Work out the finished part from the listing and answer in its coordinate system (mm). Face numbers are marked on the shaded views. A direction names the side the tool comes from. Coordinates: 2 decimals unless noted, no trailing zeros. Write each loop counter-clockwise with the first axis right and the second up, starting at its lowest first coordinate (ties: lowest second). Pieces come first, ordered by that corner, then holes. Notation, with made-up numbers: (82.25, 1) - (99.25, 1) arc R13 ccw to (99.25, 26) - close; hole circle Ø9 at (-1.75, 41.25). An arc over 180 degrees is marked (long way). Use a Markdown table: item, result. Add a question column.
(1) The part is cut by section B-B, the plane y = 40. Give the vertices of the cut face in (x, z), then the cut area to 3 significant figures.
(2) A tool of negligible diameter and unlimited length cuts with its end or side. For the marked faces 4, 5, 6 and 7, from which of +Z, -Z, +X, -X, +Y, -Y can it reach the whole face along a straight path? Write none if from no direction.
(3) The part is cut by section D-D, the plane z = 34.5. Give the vertices of the cut face in (x, y), then the cut area to 3 significant figures.
(4) Find the intervals of material crossed by line 1 (Y direction, x = 4, z = -30); line 2 (Z direction, x = 54.5, y = 61.5); line 3 (X direction, y = 60, z = -11), in increasing order. Write a range as from..to.
(5) For a pull along Y with two mould halves and no side action, classify the marked faces 1, 2 and 3 as released by +Y, released by -Y, zero draft, split by the parting line, or undercut.
(6) The part is cut by section C-C, the plane x = 24. Give the vertices of the cut face in (y, z), then the cut area to 3 significant figures.
(7) Given pin 1 Ø18.5 at (x, z) = (7.5, 30.5) entering from -Y; pin 2 Ø12 at (y, z) = (37.5, 26.5) entering from +X; pin 3 Ø13.5 at (x, z) = (6, 24) entering from +Y; pin 4 Ø10 at (x, z) = (26.5, 32) entering from -Y, each flat-ended and moving along its own axis, determine where each tip first touches the part or whether it passes through.
(8) The part is cut by section A-A, the plane z = -30. Give the vertices of the cut face in (x, y), then the cut area to 3 significant figures.
from build123d import *

# Parameters (mm, degrees)
BOSS_EXTRUDE1_DEPTH = 80
CUT_EXTRUDE1_DEPTH  = 80
SKETCH4_R           = 6
CUT_EXTRUDE4_DEPTH  = 80
BOSS_EXTRUDE2_DEPTH = 17
SKETCH9_R           = 7.5
CUT_EXTRUDE5_DEPTH  = 17
FILLET2_R           = 10
FILLET3_R           = 10


with BuildPart() as part:
    # Sketch1 → Boss-Extrude1 (new body)
    with BuildSketch(Plane(origin=(0, 0, 0), x_dir=(1, 0, 0), z_dir=(0, 1, 0))):
        Polygon((0, 0), (58, 0), (58, 13), (17, 13), (17, 47), (58, 47), (58, 60), (0, 60), align=None)
    extrude(amount=BOSS_EXTRUDE1_DEPTH)

    # Sketch2 → Cut-Extrude1 (cut)
    with BuildSketch(Plane.XY):
        with BuildLine():
            Line((38.781649875, 11), (38.781649875, 63))
            ThreePointArc((38.781649875, 63), (45, 69.218350125), (51.218350125, 63))
            Line((51.218350125, 63), (51.218350125, 11))
            ThreePointArc((51.218350125, 11), (45, 4.781649875), (38.781649875, 11))
        make_face()
    extrude(amount=-CUT_EXTRUDE1_DEPTH, mode=Mode.SUBTRACT)

    # Sketch4 → Cut-Extrude4 (cut)
    with BuildSketch(Plane(origin=(17, 0, 0), x_dir=(0, 0, -1), z_dir=(1, 0, 0))):
        with Locations((30, 18.5)):
            Circle(SKETCH4_R)
        with Locations((30, 61.5)):
            Circle(SKETCH4_R)
    extrude(amount=-CUT_EXTRUDE4_DEPTH, mode=Mode.SUBTRACT)

    # Sketch8 → Boss-Extrude2 (add)
    with BuildSketch(Plane.ZY):
        with BuildLine():
            Line((40.5, 70), (0, 70))
            Line((0, 70), (0, 10))
            Line((0, 10), (40.5, 10))
            ThreePointArc((40.5, 10), (70.5, 40), (40.5, 70))
        make_face()
    extrude(amount=-BOSS_EXTRUDE2_DEPTH)

    # Sketch9 → Cut-Extrude5 (cut)
    with BuildSketch(Plane.ZY):
        with Locations((40.5, 40)):
            Circle(SKETCH9_R)
    extrude(amount=-CUT_EXTRUDE5_DEPTH, mode=Mode.SUBTRACT)

    # Fillet2
    fillet2_edges = [part.edges().sort_by_distance(p)[0] for p in [
        (8.5, 70, 0),
    ]]
    fillet(fillet2_edges, radius=FILLET2_R - 0.0001)  # a hair under: the kernel refuses the full size

    # Fillet3
    fillet3_edges = [part.edges().sort_by_distance(p)[0] for p in [
        (8.5, 10, 0),
    ]]
    fillet(fillet3_edges, radius=FILLET3_R - 0.0001)  # a hair under: the kernel refuses the full size


solid = part.part
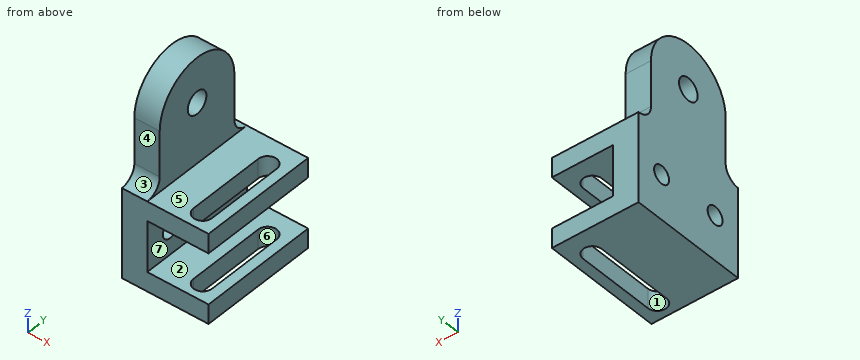
Model answer:
| question | item | result |
|---|---|---|
| 1 | outline | (0, -60) - (38.78, -60) - (38.78, -47) - (17, -47) - (17, -13) - (38.78, -13) - (38.78, 0) - (17, 0) - (17, 33) - (0, 33) - close; (0, 48) - (17, 48) - (17, 70.5) - (0, 70.5) - close; (51.22, -60) - (58, -60) - (58, -47) - (51.22, -47) - close; (51.22, -13) - (58, -13) - (58, 0) - (51.22, 0) - close |
| 1 | area | 2,710 mm^2 |
| 2 | face 4 | +Z, +X, -X, -Y |
| 2 | face 5 | +Z, +X, +Y, -Y |
| 2 | face 6 | +Z, -Z |
| 2 | face 7 | +X, +Y, -Y |
| 3 | outline | (0, 10) - (17, 10) - (17, 35.5) - (0, 35.5) - close; (0, 44.5) - (17, 44.5) - (17, 70) - (0, 70) - close |
| 3 | area | 867 mm^2 |
| 4 | line 1 | 0..12.5, 24.5..55.5, 67.5..80 |
| 4 | line 2 | -60..-47, -13..0 |
| 4 | line 3 | 0..38.78, 51.22..58 |
| 5 | face 1 | undercut |
| 5 | face 2 | zero draft |
| 5 | face 3 | released by -Y |
| 6 | outline | (0, -60) - (80, -60) - (80, -47) - (0, -47) - close; (0, -13) - (80, -13) - (80, 0) - (0, 0) - close |
| 6 | area | 2,080 mm^2 |
| 7 | pin 1 | y = 10 |
| 7 | pin 2 | x = 17 |
| 7 | pin 3 | y = 70 |
| 7 | pin 4 | through |
| 8 | outline | (0, 0) - (17, 0) - (17, 12.5) - (0, 12.5) - close; (0, 24.5) - (17, 24.5) - (17, 55.5) - (0, 55.5) - close; (0, 67.5) - (17, 67.5) - (17, 80) - (0, 80) - close |
| 8 | area | 952 mm^2 |
